```python
from build123d import *

# Parameters (mm, degrees)
SKETCH_1_W      = 7
SKETCH_1_H      = 7
EXTRUDE_1_DEPTH = 10


with BuildPart() as part:
    # 스케치1 → 보스-돌출1 (new body)
    with BuildSketch(Plane.XY):
        with BuildLine():
            Line((-3.5, 3.5), (3.5, 3.5))
            Line((3.5, 3.5), (3.5, 9.367496998))
            ThreePointArc((3.5, 9.367496998), (0, 10), (-3.5, 9.367496998))
            Line((-3.5, 9.367496998), (-3.5, 3.5))
        make_face()
        with BuildLine():
            Line((-9.367496998, -3.5), (-3.5, -3.5))
            Line((-3.5, -3.5), (-3.5, 3.5))
            Line((-3.5, 3.5), (-9.367496998, 3.5))
            ThreePointArc((-9.367496998, 3.5), (-10, 0), (-9.367496998, -3.5))
        make_face()
        Rectangle(SKETCH_1_W, SKETCH_1_H)
        with BuildLine():
            ThreePointArc((-3.5, -9.367496998), (-1.778346145, -9.840603893), (0, -10))
            ThreePointArc((0, -10), (1.778346145, -9.840603893), (3.5, -9.367496998))
            Line((3.5, -9.367496998), (3.5, -3.5))
            Line((3.5, -3.5), (-3.5, -3.5))
            Line((-3.5, -3.5), (-3.5, -9.367496998))
        make_face()
        with BuildLine():
            Line((3.5, 3.5), (3.5, -3.5))
            Line((3.5, -3.5), (9.367496998, -3.5))
            ThreePointArc((9.367496998, -3.5), (9.840603893, -1.778346145), (10, 0))
            ThreePointArc((10, 0), (9.840603893, 1.778346145), (9.367496998, 3.5))
            Line((9.367496998, 3.5), (3.5, 3.5))
        make_face()
    extrude(amount=EXTRUDE_1_DEPTH)


solid = part.part
```
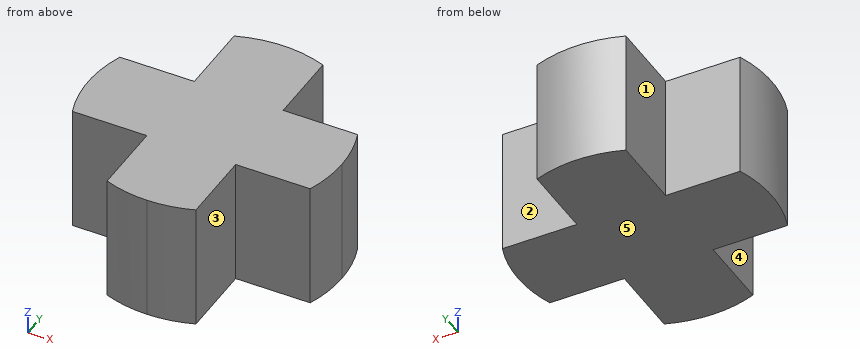
Input: part model. Units: mm. Frame: model coordinates. Face numbers are marked on the shaded views. A direction names the side the tool comes from. Round coordinates to 2 decimals unless told otherwise and drop trailing zeros. Loops run counter-clockwise (first coordinate to the right, second up) from the corner with the lowest first, then second, coordinate; pieces in that order, holes last.
1) Section query A-A on z = 3.5. Return the cut outline in (x, y).
Ans:
outline: (-9.37, -3.5) - (-3.5, -3.5) - (-3.5, -9.37) arc R10 ccw to (3.5, -9.37) - (3.5, -3.5) - (9.37, -3.5) arc R10 ccw to (9.37, 3.5) - (3.5, 3.5) - (3.5, 9.37) arc R10 ccw to (-3.5, 9.37) - (-3.5, 3.5) - (-9.37, 3.5) arc R10 ccw to start
2) Pin query (flat end, axial travel): pin 1 (3 mm diameter, centred on x = 6, z = 4, fed in from -Y); pin 2 (1.8 mm diameter, centred on y = 5.5, z = 5, fed in from -X); pin 3 (4 mm diameter, centred on y = -3.5, z = 8, fed in from -X). Return the tip coordinate at first contact, or that it passes through.
Ans:
pin 1: stops at y = -3.5
pin 2: stops at x = -3.5
pin 3: stops at x = -9.89
3) Section query B-B on y = 6.5. Return the cut outline in (x, z), plus the area to 3 significant figures.
Ans:
outline: (-3.5, 0) - (3.5, 0) - (3.5, 10) - (-3.5, 10) - close
area: 70.0 mm2
4) Material intervals for line 1 (Y direction, x = 6.25, z = 9.25); line 2 (X direction, y = 0.25, z = 5), sorted ascending.
Ans:
line 1: y = -3.5 to 3.5
line 2: x = -10 to 10
5) Set-up query: the marked faces 1, 2, 3, 4 and 5. Return all of +Z, -Z, +X, -X, +Y, -Y with unobstructed straight access to the full face (end or side cutting, diameter ignored); none if empty.
Ans:
face 1: +Z, -Z, -X, +Y
face 2: +Z, -Z, +X, +Y
face 3: +Z, -Z, +X, -Y
face 4: +Z, -Z, -X, -Y
face 5: -Z, +X, -X, +Y, -Y
